Read the model definition and answer for the solid it produces. Units are mm, in the model's axes. Give positions to 0.01 mm unless a question says otherwise; leave off trailing zeros. Loops run counter-clockwise (first coordinate to the right, second up) from the corner with the lowest first, then second, coordinate; pieces in that order, holes last.
(1) Find section A-A, the plane x = -9. Write down the section's boundary in (y, z), then the cut area to 3 significant figures.
(2) Find section C-C, the plane z = 2. Write down the section's boundary in (x, y).
(3) Straight lines are drawn through the part: probe 1 along Z at (x, y) = (-60, 2.7); probe 2 along X at (y, z) = (0.25, -7.5); probe 3 along Y at (x, z) = (-88, -6.5). For each, find the intervals that lie inside material, in ascending order.
(4) Determine the mould class of faces 1 (the face through (0, 3, -19)), 2 (the face through (-1, 0, 0)) for opening direction Z: pulls with the +Z half, pulls with the -Z half, needs draft (parallel to the pull), parting line crosses it, or undercut.
(5) Find section B-B, the plane y = 1. Write down the section's boundary in (x, z), then the cut area to 3 significant figures.
(6) Each of these flat-tipped pins is pushed along its axis until it touches: P1, Ø1.5, axis at y = 1, z = 13.5, coming from the -X side; P2, Ø1.5, axis at y = 1, z = -4, coming from the +X side; P3, Ø1.5, axis at x = -18.5, y = 1.5, coming from the -Z side. Where does it stop, or does it pass through?
```python
from build123d import *

# Parameters (mm, degrees)
SKETCH_228_W        = 210
SKETCH_228_H        = 53
EXTRUDE_1_DEPTH     = 50
SKETCH_3_W          = 200
SKETCH_3_H          = 43
CUT_EXTRUDE_1_DEPTH = 45
SKETCH_4_R          = 3.5
EXTRUDE_2_DEPTH     = 2
EXTRUDE_2_TAPER     = 1
FILLET_2_R          = 0.5
SKETCH_4_5_R        = 3.5
EXTRUDE_3_DEPTH     = 2
SKETCH_4_6_R        = 3.5
EXTRUDE_4_DEPTH     = 2
SKETCH_4_7_R        = 3.5
EXTRUDE_5_DEPTH     = 2
FILLET_3_R          = 0.5
FILLET_4_R          = 0.5
FILLET_5_R          = 0.5
SKETCH_7_R          = 6
CUT_EXTRUDE_2_DEPTH = 14
CUT_EXTRUDE_2_DRAFT = -5
FILLET_6_R          = 2
SKETCH_8_R          = 7
EXTRUDE_6_DEPTH     = 7
EXTRUDE_6_TAPER     = 5
SKETCH_9_R          = 5.15
CUT_EXTRUDE_3_DEPTH = 7
CUT_EXTRUDE_3_DRAFT = 5
SKETCH_10_W         = 29.4
SKETCH_10_H         = 26.3
CUT_EXTRUDE_4_DEPTH = 5
SKETCH_13_W         = 39.2
SKETCH_13_H         = 27.5
CUT_EXTRUDE_5_DEPTH = 2
SKETCH_14_W         = 6
SKETCH_14_H         = 6
CUT_EXTRUDE_6_DEPTH = 5
FILLET_7_R          = 2
EXTRUDE_8_DEPTH     = 3
SKETCH_18_W         = 200
SKETCH_18_H         = 43
SKETCH_18_W_2       = 194
SKETCH_18_H_2       = 37
EXTRUDE_4681_DEPTH  = 3
SKETCH_21_W         = 4.1
SKETCH_21_H         = 2.2
CUT_EXTRUDE_7_DEPTH = 3


with BuildPart() as part:
    # Sketch 228 → Бобышка-Вытянуть1 (new body)
    with BuildSketch(Plane(origin=(0, 0, 0), x_dir=(1, 0, 0), z_dir=(0, 1, 0))):
        Rectangle(SKETCH_228_W, SKETCH_228_H)
    extrude(amount=EXTRUDE_1_DEPTH)

    # Эскиз3 → Вырез-Вытянуть1 (cut)
    with BuildSketch(Plane.XZ):
        Rectangle(SKETCH_3_W, SKETCH_3_H)
    extrude(amount=-CUT_EXTRUDE_1_DEPTH, mode=Mode.SUBTRACT)

    # Эскиз4 → Бобышка-Вытянуть2 (add)
    with BuildSketch(Plane(origin=(0, 50, 0), x_dir=(1, 0, 0), z_dir=(0, 1, 0))):
        with Locations((98, 19.5)):
            Circle(SKETCH_4_R)
    extrude(amount=EXTRUDE_2_DEPTH, taper=EXTRUDE_2_TAPER)

    # Скругление2
    fillet_2_edges = [part.edges().sort_by_distance(p)[0] for p in [
        (94.53491013, 52, -19.5),
    ]]
    fillet(fillet_2_edges, radius=FILLET_2_R)

    # Эскиз4<5> → Бобышка-Вытянуть3 (add)
    with BuildSketch(Plane(origin=(0, 50, 0), x_dir=(1, 0, 0), z_dir=(0, 1, 0))):
        with Locations(Location((98, -19.5, 0), (0, 0, 90))):
            Circle(SKETCH_4_5_R)
    extrude(amount=EXTRUDE_3_DEPTH)

    # Эскиз4<6> → Бобышка-Вытянуть4 (add)
    with BuildSketch(Plane(origin=(0, 50, 0), x_dir=(1, 0, 0), z_dir=(0, 1, 0))):
        with Locations(Location((-98, -19.5, 0), (0, 0, 270))):
            Circle(SKETCH_4_6_R)
    extrude(amount=EXTRUDE_4_DEPTH)

    # Эскиз4<7> → Бобышка-Вытянуть5 (add)
    with BuildSketch(Plane(origin=(0, 50, 0), x_dir=(1, 0, 0), z_dir=(0, 1, 0))):
        with Locations(Location((-98, 19.5, 0), (0, 0, 90))):
            Circle(SKETCH_4_7_R)
    extrude(amount=EXTRUDE_5_DEPTH)

    # Скругление3
    fillet_3_edges = [part.edges().sort_by_distance(p)[0] for p in [
        (-98, 52, 16),
    ]]
    fillet(fillet_3_edges, radius=FILLET_3_R)

    # Скругление4
    fillet_4_edges = [part.edges().sort_by_distance(p)[0] for p in [
        (-98, 52, -16),
    ]]
    fillet(fillet_4_edges, radius=FILLET_4_R)

    # Скругление5
    fillet_5_edges = [part.edges().sort_by_distance(p)[0] for p in [
        (98, 52, 23),
    ]]
    fillet(fillet_5_edges, radius=FILLET_5_R)


with BuildPart() as cut_extrude_2_tool:
    # Эскиз7 → Вырез-Вытянуть2 (with draft: the straight prism first)
    with BuildSketch(Plane(origin=(0, 0, -26.5), x_dir=(-1, 0, 0), z_dir=(0, 0, -1))):
        with Locations((0, 35.081888724)):
            Circle(SKETCH_7_R)
    extrude(amount=-CUT_EXTRUDE_2_DEPTH)
    # Вырез-Вытянуть2: the draft: its side faces are tilted about the plane it starts from
    cut_extrude_2_sides = [cut_extrude_2_tool.faces().sort_by_distance(p)[0] for p in [
        (6, 35.081888724, -19.5),
    ]]
    draft(cut_extrude_2_sides, Plane(origin=(0, 0, -26.5), x_dir=(-1, 0, 0), z_dir=(0, 0, -1)), CUT_EXTRUDE_2_DRAFT)


with BuildPart() as part_1:
    add(part.part)

    # Вырез-Вытянуть2: cut by cut_extrude_2_tool
    add(cut_extrude_2_tool.part, mode=Mode.SUBTRACT)

    # Скругление6
    fillet_6_edges = [part_1.edges().sort_by_distance(p)[0] for p in [
        (6, 35.081888724, -26.5),
    ]]
    fillet(fillet_6_edges, radius=FILLET_6_R)

    # Эскиз8 → Бобышка-Вытянуть6 (add)
    with BuildSketch(Plane.XY.offset(-21.5)):
        with Locations((0, 35.081888724)):
            Circle(SKETCH_8_R)
    extrude(amount=EXTRUDE_6_DEPTH, taper=EXTRUDE_6_TAPER)


with BuildPart() as cut_extrude_3_tool:
    # Эскиз9 → Вырез-Вытянуть3 (with draft: the straight prism first)
    with BuildSketch(Plane.XY.offset(-14.5)):
        with Locations((0, 35.081888724)):
            Circle(SKETCH_9_R)
    extrude(amount=-CUT_EXTRUDE_3_DEPTH)
    # Вырез-Вытянуть3: the draft: its side faces are tilted about the plane it starts from
    cut_extrude_3_sides = [cut_extrude_3_tool.faces().sort_by_distance(p)[0] for p in [
        (-5.15, 35.081888724, -18),
    ]]
    draft(cut_extrude_3_sides, Plane.XY.offset(-14.5), CUT_EXTRUDE_3_DRAFT)


with BuildPart() as part_2:
    add(part_1.part)

    # Вырез-Вытянуть3: cut by cut_extrude_3_tool
    add(cut_extrude_3_tool.part, mode=Mode.SUBTRACT)

    # Эскиз10 → Вырез-Вытянуть4 (cut)
    with BuildSketch(Plane.XY.offset(26.5)):
        with Locations((-50, 25)):
            Rectangle(SKETCH_10_W, SKETCH_10_H)
    extrude(amount=-CUT_EXTRUDE_4_DEPTH, mode=Mode.SUBTRACT)

    # Эскиз13 → Вырез-Вытянуть5 (cut)
    with BuildSketch(Plane(origin=(0, 0, 21.5), x_dir=(-1, 0, 0), z_dir=(0, 0, -1))):
        with Locations((50, 25)):
            Rectangle(SKETCH_13_W, SKETCH_13_H)
    extrude(amount=-CUT_EXTRUDE_5_DEPTH, mode=Mode.SUBTRACT)

    # Эскиз14 → Вырез-Вытянуть6 (cut)
    with BuildSketch(Plane.XY.offset(26.5)):
        with Locations((-76.5, 31.8)):
            Rectangle(SKETCH_14_W, SKETCH_14_H)
        with Locations((-76.5, 18.2)):
            Rectangle(SKETCH_14_W, SKETCH_14_H)
    extrude(amount=-CUT_EXTRUDE_6_DEPTH, mode=Mode.SUBTRACT)

    # Скругление7
    fillet_7_edges = [part_2.edges().sort_by_distance(p)[0] for p in [
        (-105, 50, 0),
        (0, 50, 26.5),
        (105, 50, 0),
        (105, 25, 26.5),
        (-105, 25, 26.5),
        (-105, 25, -26.5),
        (105, 25, -26.5),
        (0, 50, -26.5),
    ]]
    fillet(fillet_7_edges, radius=FILLET_7_R)


with BuildPart() as body_2:
    # Эскиз17 → Бобышка-Вытянуть8 (new body)
    with BuildSketch(Plane.XZ):
        with BuildLine():
            Line((-105, 24.5), (-105, -24.5))
            ThreePointArc((-105, -24.5), (-104.414213562, -25.914213562), (-103, -26.5))
            Line((-103, -26.5), (103, -26.5))
            ThreePointArc((103, -26.5), (104.414213562, -25.914213562), (105, -24.5))
            Line((105, -24.5), (105, 24.5))
            ThreePointArc((105, 24.5), (104.414213562, 25.914213562), (103, 26.5))
            Line((103, 26.5), (-103, 26.5))
            ThreePointArc((-103, 26.5), (-104.414213562, 25.914213562), (-105, 24.5))
        make_face()
    extrude(amount=EXTRUDE_8_DEPTH)

    # Эскиз18 → Extrude 4681 (add)
    with BuildSketch(Plane(origin=(0, 0, 0), x_dir=(1, 0, 0), z_dir=(0, 1, 0))):
        Rectangle(SKETCH_18_W, SKETCH_18_H)
        Rectangle(SKETCH_18_W_2, SKETCH_18_H_2, mode=Mode.SUBTRACT)
    extrude(amount=EXTRUDE_4681_DEPTH)

    # Эскиз21 → Вырез-Вытянуть7 (cut)
    with BuildSketch(Plane.XZ.offset(3)):
        with Locations((10.5, 16.9)):
            Rectangle(SKETCH_21_W, SKETCH_21_H)
        with Locations((18.5, 16.9)):
            Rectangle(SKETCH_21_W, SKETCH_21_H)
    extrude(amount=-CUT_EXTRUDE_7_DEPTH, mode=Mode.SUBTRACT)


solid = body_2.part
```
Entries:
1. outline: (-3, -26.5) - (0, -26.5) - (0, -21.5) - (3, -21.5) - (3, -18.5) - (0, -18.5) - (0, 18.5) - (3, 18.5) - (3, 21.5) - (0, 21.5) - (0, 26.5) - (-3, 26.5) - close
1. area: 177 mm2
2. outline: (-105, -3) - (105, -3) - (105, 0) - (100, 0) - (100, 3) - (97, 3) - (97, 0) - (-97, 0) - (-97, 3) - (-100, 3) - (-100, 0) - (-105, 0) - close
3. probe 1: z = -21.5 to -18.5, 18.5 to 21.5
3. probe 2: x = -100 to -97, 97 to 100
3. probe 3: y = -3 to 0
4. face 1: needs draft
4. face 2: undercut
5. outline: (-100, -21.5) - (100, -21.5) - (100, 21.5) - (-100, 21.5) - close; hole (-97, -18.5) - (97, -18.5) - (97, 18.5) - (-97, 18.5) - close
5. area: 1,420 mm2
6. P1: stops at x = -100
6. P2: stops at x = 100
6. P3: stops at z = -21.5
